Design review of the part shown in the three views and the two pictorial views. Dimensions are in mm from the part's minimum x, y and z. A direction names the side the tool comes from. Coordinates: 2 decimals unless noted, no trailing zeros. Loops run counter-clockwise (first coordinate to the right, second up) from the corner with the lowest first, then second, coordinate; pieces in that order, holes last. Notation, with made-up numbers: M 16,49 L 50,49 A31 cw 50,87 Z; hole C 29,71 d7. An arc over 180 degrees is marked long. Answer as a JSON object with one key per item and string values. Group by question number.
Item 1: Insertion check: pin 1 (2.5 mm diameter, centred on x = 24, z = 6, fed in from -Y); pin 2 (3 mm diameter, centred on y = 2.5, z = 4, fed in from -X). Each pin has a flat end and moves straight along its axis. Give the tip position at first contact, or say it passes through.
Item 2: Add section A-A (z = 2.5). State the section outline as (x, y) points.
Item 3: Wall thickness on L1, parallel to X at y = 9, z = 9; L2, parallel to Y at x = 26.5, z = 3: over which ranges is each line inside the solid? List them lowest first. Write a range as from..to.
Item 4: Add section B-B (x = 27.5). State the section outline as (y, z) points.
Item 5: Tool access review of the marked faces 1, 2 and 3: name each direction out of +Z, -Z, +X, -X, +Y, -Y from which nothing blocks a thin tool from reaching the whole face with its end or side.
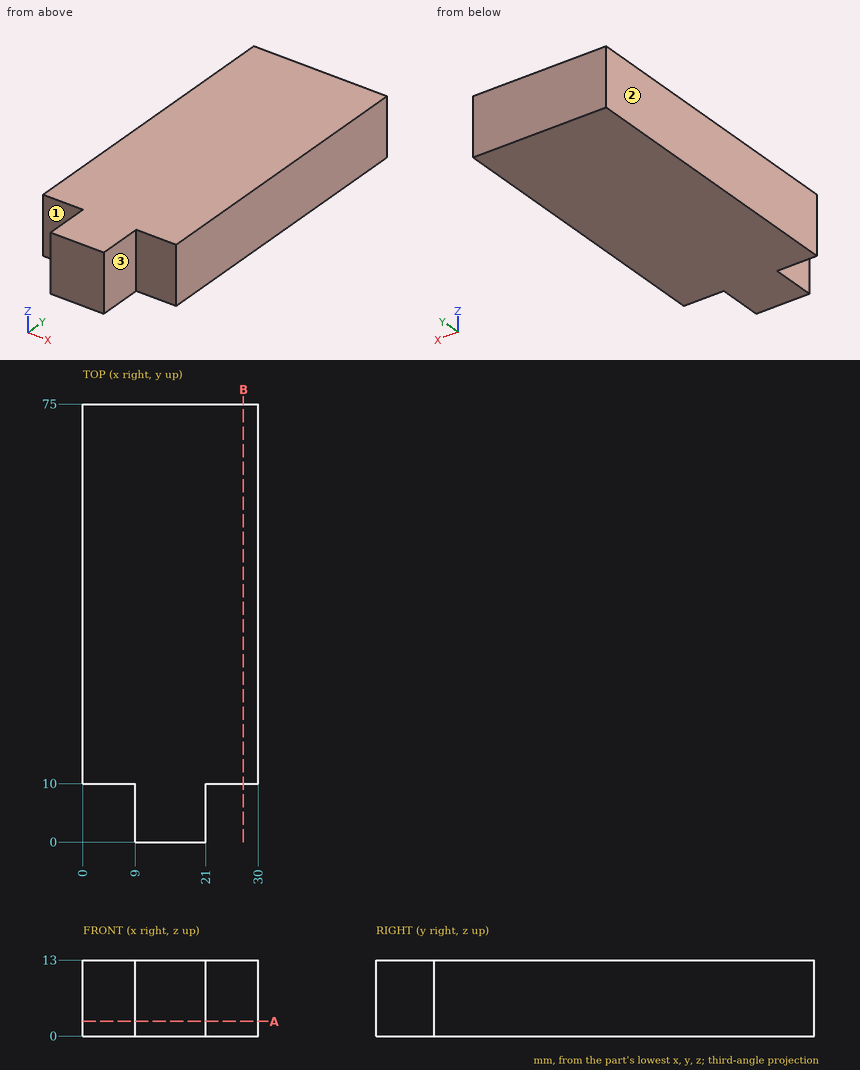
From the geometry:
{
 "1": {"pin 1": "stops at y = 10", "pin 2": "stops at x = 9"},
 "2": {"outline": "M 0,10 L 9,10 L 9,0 L 21,0 L 21,10 L 30,10 L 30,75 L 0,75 Z"},
 "3": {"L1": "x = 9..21", "L2": "y = 10..75"},
 "4": {"outline": "M 10,0 L 75,0 L 75,13 L 10,13 Z"},
 "5": {"face 1": "+Z, -Z, -X, -Y", "face 2": "+Z, -Z, -X, +Y, -Y", "face 3": "+Z, -Z, +X, -Y"}
}
